The model under review builds one solid part; all positions refer to its coordinate system, in mm. A direction names the side the tool comes from. Round coordinates to 2 decimals unless told otherwise and drop trailing zeros. Write each loop counter-clockwise with the first axis right and the second up, starting at its lowest first coordinate (ties: lowest second). Pieces come first, ordered by that corner, then holes. Notation, with made-up numbers: (-11, -2) -> (33, -2) arc R14 ccw to (33, 15) -> close; hole circle Ø9 at (-35, 19.25). An arc over 180 degrees is marked (long way). Answer as a JSON object with one key per item and string values. Group by question number.
1) Machinability: for faces 4 (the flat face through (29, -17, 0)), 5 (the flat face through (29, -17, 3)), 6 (the cylindrical face through (0, -34, 3)), which of the approach directions +Z, -Z, +X, -X, +Y, -Y give a long, thin tool a straight path to every point of the face, cutting with its end or side? Answer none if there is none.
2) We need section C-C, the plane y = 17.5. Write out the cut boundary in (x, z).
3) Insertion check: pin 1 Ø1 at (y, z) = (33, 1.5) entering from +X; pin 2 Ø1.5 at (x, z) = (5.5, 2.5) entering from -Y; pin 3 Ø0.6 at (y, z) = (33, 1.5) entering from -X. Each pin has a flat end and moves straight along its axis. Give the tip position at first contact, or say it passes through.
4) To check wall thickness, follow probe 1 along Y at (x, z) = (-29, 2); probe 2 along X at (y, z) = (-21, 1); probe 3 along Y at (x, z) = (6, 5.25). State the ranges of each line that lie inside material, in increasing order. Write a range as [from, to].
5) Mouldability with a two-part tool opening along Y and no side actions: class faces 1 (the flat face through (-29, -17, 3)), 2 (the flat face through (-12, 32, 7)), 3 (the cylindrical face through (-5.077, 38.668, 3.451)) as pulls with the +Y half, pulls with the -Y half, needs draft (parallel to the pull), parting line crosses it, or undercut.
6) We need section D-D, the plane z = 1. Write out the cut boundary in (x, y).
7) We need section B-B, the plane z = 5. Write out the cut boundary in (x, y).
8) We need section A-A, the plane x = 0. Write out the cut boundary in (y, z), then the cut area to 3 significant figures.
from build123d import *

# Parameters (mm, degrees)
F0_R     = 39
F1_DEPTH = 7
F2_DEPTH = 3
F3_DEPTH = 3
F4_DEPTH = 3


with BuildPart() as f1:
    # F0 (on Top) → F1 (new body)
    with BuildSketch(Plane.XY):
        Circle(F0_R)
        with BuildLine():
            ThreePointArc((4, 33.763886), (25.41653, 22.58318), (34, 0))
            ThreePointArc((34, 0), (33.30295, -6.849342), (31.240383, -13.417841))
            ThreePointArc((31.240383, -13.417841), (29.444864, -17), (27.240383, -20.346045))
            ThreePointArc((27.240383, -20.346045), (0, -34), (-27.240383, -20.346045))
            ThreePointArc((-27.240383, -20.346045), (-29.444864, -17), (-31.240383, -13.417841))
            ThreePointArc((-31.240383, -13.417841), (-29.444864, 17), (-4, 33.763886))
            ThreePointArc((-4, 33.763886), (0, 34), (4, 33.763886))
        make_face(mode=Mode.SUBTRACT)
    extrude(amount=F1_DEPTH)

    # F0 (on Top) → F2 (join)
    with BuildSketch(Plane.XY):
        with BuildLine():
            Line((4, 32.5), (4, 33.763886))
            ThreePointArc((4, 33.763886), (0, 34), (-4, 33.763886))
            Line((-4, 33.763886), (-4, 32.5))
            Line((-4, 32.5), (4, 32.5))
        make_face()
    extrude(amount=F2_DEPTH)

    # F0 (on Top) → F3 (join)
    with BuildSketch(Plane.XY):
        with BuildLine():
            ThreePointArc((27.240383, -20.346045), (29.444864, -17), (31.240383, -13.417841))
            Line((31.240383, -13.417841), (30.145826, -12.785898))
            Line((30.145826, -12.785898), (26.145826, -19.714102))
            Line((26.145826, -19.714102), (27.240383, -20.346045))
        make_face()
    extrude(amount=F3_DEPTH)

    # F0 (on Top) → F4 (join)
    with BuildSketch(Plane.XY):
        with BuildLine():
            Line((-30.145826, -12.785898), (-31.240383, -13.417841))
            ThreePointArc((-31.240383, -13.417841), (-29.444864, -17), (-27.240383, -20.346045))
            Line((-27.240383, -20.346045), (-26.145826, -19.714102))
            Line((-26.145826, -19.714102), (-30.145826, -12.785898))
        make_face()
    extrude(amount=F4_DEPTH)


solid = f1.part
Here are the results:
{
 "1": {"face 4": "-Z, +X, -X, +Y, -Y", "face 5": "+Z", "face 6": "+Z, -Z"},
 "2": {"outline": "(-34.85, 0) -> (-29.15, 0) -> (-29.15, 7) -> (-34.85, 7) -> close; (29.15, 0) -> (34.85, 0) -> (34.85, 7) -> (29.15, 7) -> close"},
 "3": {"pin 1": "stops at x = 21.56", "pin 2": "stops at y = -38.71", "pin 3": "stops at x = -21.25"},
 "4": {"probe 1": "y = [-26.08, -14.77], [17.75, 26.08]", "probe 2": "x = [-32.86, -26.74], [26.74, 32.86]", "probe 3": "y = [-38.54, -33.47], [33.47, 38.54]"},
 "5": {"face 1": "undercut", "face 2": "needs draft", "face 3": "parting line crosses it"},
 "6": {"outline": "circle Ø78 at (0, 0); hole (-31.24, -13.42) -> (-30.15, -12.79) -> (-26.15, -19.71) -> (-27.24, -20.35) arc R34 ccw to (27.24, -20.35) -> (26.15, -19.71) -> (30.15, -12.79) -> (31.24, -13.42) arc R34 ccw to (34, 0) arc R34 ccw to (4, 33.76) -> (4, 32.5) -> (-4, 32.5) -> (-4, 33.76) arc R34 ccw to start"},
 "7": {"outline": "circle Ø78 at (0, 0); hole (-31.24, -13.42) arc R34 ccw to (-27.24, -20.35) arc R34 ccw to (27.24, -20.35) arc R34 ccw to (31.24, -13.42) arc R34 ccw to (34, 0) arc R34 ccw to (4, 33.76) arc R34 ccw to (-4, 33.76) arc R34 ccw to start"},
 "8": {"outline": "(-39, 0) -> (-34, 0) -> (-34, 7) -> (-39, 7) -> close; (32.5, 0) -> (39, 0) -> (39, 7) -> (34, 7) -> (34, 3) -> (32.5, 3) -> close", "area": "74.5 mm^2"}
}
